from build123d import *

# Parameters (mm, degrees)
ESTRUSIONE_ESTRUSIONE1_DEPTH = 20
TAGLIO_ESTRUSIONE1_REACH     = 37.979
ESTRUSIONE_ESTRUSIONE4_DEPTH = 0.6
SCHIZZO12_W                  = 2
SCHIZZO12_H                  = 6
TAGLIO_ESTRUSIONE2_DEPTH     = 11


with BuildPart() as part:
    # Schizzo2 → Estrusione-Estrusione1 (new body)
    with BuildSketch(Plane.XY):
        with BuildLine():
            Line((-4, 9.5), (-11, 9.5))
            Line((-11, 9.5), (-11, 23.5))
            Line((-11, 23.5), (-6, 23.5))
            ThreePointArc((-6, 23.5), (-5.292893219, 23.207106781), (-5, 22.5))
            Line((-5, 22.5), (-5, 12.5))
            Line((-5, 12.5), (4, 12.5))
            Line((4, 12.5), (4, 9.5))
            Line((4, 9.5), (4, 6.5))
            Line((4, 6.5), (7.5, 6.5))
            Line((7.5, 6.5), (7.5, 4))
            Line((7.5, 4), (4, 0))
            Line((4, 0), (-4, 0))
            Line((-4, 0), (-7.5, 4))
            Line((-7.5, 4), (-7.5, 6.5))
            Line((-7.5, 6.5), (-4, 6.5))
            Line((-4, 6.5), (-4, 9.5))
        make_face()
    extrude(amount=-ESTRUSIONE_ESTRUSIONE1_DEPTH)

    # Schizzo6 → Taglio-Estrusione1 (cut, up to next)
    with BuildSketch(Plane.ZY.offset(11), mode=Mode.PRIVATE) as taglio_estrusione1_sk1:
        with BuildLine():
            Line((-8.5, 20), (-8.5, 17))
            ThreePointArc((-8.5, 17), (-10, 15.5), (-11.5, 17))
            Line((-11.5, 17), (-11.5, 20))
            ThreePointArc((-11.5, 20), (-10, 21.5), (-8.5, 20))
        make_face()
    taglio_estrusione1_tool1 = extrude(taglio_estrusione1_sk1.sketch, amount=-TAGLIO_ESTRUSIONE1_REACH, mode=Mode.PRIVATE) & part.part
    add(taglio_estrusione1_tool1.solids().sort_by_distance((-11, 18.5, -10))[0], mode=Mode.SUBTRACT)

    # Schizzo11 → Estrusione-Estrusione4 (add)
    with BuildSketch(Plane(origin=(0, 0, -20), x_dir=(-1, 0, 0), z_dir=(0, 0, -1))):
        with BuildLine():
            Line((-1.916666667, 6), (-2.5, 6))
            add(Edge.make_bspline(
                [(-2.5, 6), (-2.484196549, 6.065431756), (-2.453302094, 6.193345487), (-2.388863743, 6.376101829), (-2.318665127, 6.549045511), (-2.234371075, 6.708938219), (-2.142426246, 6.858993324), (-2.037084049, 6.995807413), (-1.923204564, 7.122860063), (-1.797243944, 7.235613218), (-1.665147858, 7.337714716), (-1.525054993, 7.424768393), (-1.379783905, 7.499656106), (-1.228328086, 7.561350822), (-1.070236625, 7.607826795), (-0.906938753, 7.641546577), (-0.738006538, 7.66344436), (-0.623332441, 7.665581492), (-0.565104167, 7.666666667)],
                knots=[0, 0, 0, 0, 1.162005537, 2.271625781, 3.343758855, 4.383309926, 5.390229558, 6.379919256, 7.361854164, 8.333198761, 9.295911338, 10.242430842, 11.177959212, 12.116337295, 13.062827104, 14.020064771, 14.994644689, 16, 16, 16, 16], degree=3))
            add(Edge.make_bspline(
                [(-0.565104167, 7.666666667), (-0.480264789, 7.664105239), (-0.312436625, 7.659038256), (-0.065876681, 7.612768588), (0.171887412, 7.539550485), (0.398253158, 7.438384992), (0.608515961, 7.313608553), (0.795597451, 7.165102613), (0.956961828, 6.995732482), (1.092337101, 6.80865772), (1.198333527, 6.608726059), (1.276493935, 6.402954339), (1.324077057, 6.191830678), (1.330243806, 6.049281445), (1.333333333, 5.977864583)],
                knots=[0, 0, 0, 0, 1.083050992, 2.142477498, 3.193116406, 4.255571735, 5.30263384, 6.308962982, 7.297363603, 8.282367274, 9.249857812, 10.179914175, 11.08814088, 12, 12, 12, 12], degree=3))
            add(Edge.make_bspline(
                [(1.333333333, 5.977864583), (1.331172379, 5.909137679), (1.326943725, 5.774649792), (1.291038272, 5.578309869), (1.230613784, 5.393261183), (1.146912796, 5.218724739), (1.038564203, 5.055807179), (0.907314909, 4.904141953), (0.752238537, 4.763056374), (0.634720509, 4.682234495), (0.57421875, 4.640625)],
                knots=[0, 0, 0, 0, 1.024540389, 2.004866551, 2.965041327, 3.920577974, 4.882998113, 5.874504559, 6.905732034, 8, 8, 8, 8], degree=3))
            add(Edge.make_bspline(
                [(0.57421875, 4.640625), (0.643363437, 4.607236967), (0.780359061, 4.541085617), (0.967095758, 4.411353496), (1.136611813, 4.261563137), (1.231147291, 4.144669639), (1.278645833, 4.0859375)],
                knots=[0, 0, 0, 0, 1.015518401, 2.012035669, 3.001164323, 4, 4, 4, 4], degree=3))
            add(Edge.make_bspline(
                [(1.278645833, 4.0859375), (1.309922612, 4.043115961), (1.37196399, 3.958174116), (1.448544267, 3.821606468), (1.518018337, 3.683525131), (1.572154458, 3.540229091), (1.614077354, 3.393379209), (1.644044271, 3.24272333), (1.662660533, 3.088138431), (1.665326558, 2.983558111), (1.666666667, 2.930989583)],
                knots=[0, 0, 0, 0, 1.025084078, 2.033381695, 3.024893161, 4.013698104, 4.991890475, 5.976764909, 6.982997093, 8, 8, 8, 8], degree=3))
            add(Edge.make_bspline(
                [(1.666666667, 2.930989583), (1.663333999, 2.83997153), (1.656684346, 2.658363755), (1.597248208, 2.390053558), (1.505109333, 2.127777625), (1.374260737, 1.876924352), (1.214792507, 1.64221793), (1.025071762, 1.43221907), (0.807254146, 1.251707377), (0.56432937, 1.100888382), (0.301140417, 0.980326526), (0.019642889, 0.896648418), (-0.276107211, 0.842148704), (-0.478920764, 0.836304519), (-0.58203125, 0.833333333)],
                knots=[0, 0, 0, 0, 0.955779014, 1.907060117, 2.875433937, 3.871313158, 4.872415639, 5.851225146, 6.836215519, 7.83643374, 8.849228613, 9.86973379, 10.916971861, 12, 12, 12, 12], degree=3))
            add(Edge.make_bspline(
                [(-0.58203125, 0.833333333), (-0.651524236, 0.834945729), (-0.78826326, 0.838118387), (-0.9892869, 0.859807218), (-1.181170056, 0.899420085), (-1.364172166, 0.952726223), (-1.538455805, 1.020310887), (-1.703489143, 1.104474184), (-1.860287517, 1.203481259), (-2.007371283, 1.318500779), (-2.144722909, 1.447166124), (-2.268692254, 1.591761428), (-2.381346155, 1.74961375), (-2.479668199, 1.922556569), (-2.568136825, 2.108354904), (-2.640901459, 2.309387829), (-2.704946086, 2.523858156), (-2.73472252, 2.673316816), (-2.75, 2.75)],
                knots=[0, 0, 0, 0, 1.048658725, 2.063410685, 3.046034179, 4.001477787, 4.936774919, 5.862367409, 6.792675028, 7.730719943, 8.675894397, 9.627829632, 10.600096036, 11.597688215, 12.626045268, 13.701542398, 14.82072376, 16, 16, 16, 16], degree=3))
            Line((-2.75, 2.75), (-2.166666667, 2.75))
            add(Edge.make_bspline(
                [(-2.166666667, 2.75), (-2.151469125, 2.699951833), (-2.121908588, 2.602603799), (-2.071590606, 2.462500375), (-2.014263815, 2.33406399), (-1.952765349, 2.216352478), (-1.888176806, 2.108206588), (-1.815906231, 2.012485974), (-1.74130639, 1.924986312), (-1.685073305, 1.875689176), (-1.657552083, 1.8515625)],
                knots=[0, 0, 0, 0, 1.198163088, 2.33053128, 3.407730985, 4.417276592, 5.372219308, 6.28897303, 7.162600585, 8, 8, 8, 8], degree=3))
            add(Edge.make_bspline(
                [(-1.657552083, 1.8515625), (-1.621158441, 1.823504166), (-1.548483496, 1.767474107), (-1.430056781, 1.695971082), (-1.305507707, 1.634014892), (-1.172137598, 1.586688029), (-1.032824452, 1.54661523), (-0.885316488, 1.520391409), (-0.730915085, 1.502399091), (-0.625489239, 1.500811361), (-0.571614583, 1.5)],
                knots=[0, 0, 0, 0, 0.946170439, 1.889420265, 2.845303464, 3.807233317, 4.801018734, 5.828864929, 6.890507805, 8, 8, 8, 8], degree=3))
            add(Edge.make_bspline(
                [(-0.571614583, 1.5), (-0.51078665, 1.501143824), (-0.391842877, 1.503380473), (-0.218283853, 1.523949643), (-0.053170021, 1.553906125), (0.101665412, 1.600173093), (0.24825064, 1.657337532), (0.384530847, 1.729113142), (0.512295044, 1.813324768), (0.629906797, 1.909040348), (0.735662739, 2.013823125), (0.828778978, 2.123418828), (0.907939064, 2.237365369), (0.97179428, 2.356293307), (1.022216731, 2.479710161), (1.056542675, 2.607962273), (1.080409774, 2.740000053), (1.082353483, 2.829753852), (1.083333333, 2.875)],
                knots=[0, 0, 0, 0, 1.217147791, 2.380027433, 3.494444702, 4.572153297, 5.609568379, 6.639424714, 7.649109417, 8.668170816, 9.669597737, 10.625200337, 11.543417969, 12.441394052, 13.322311151, 14.205496177, 15.095365482, 16, 16, 16, 16], degree=3))
            add(Edge.make_bspline(
                [(1.083333333, 2.875), (1.080491345, 2.935563915), (1.074821509, 3.056390388), (1.031534147, 3.234151597), (0.960333399, 3.405423649), (0.860655878, 3.567284402), (0.739318097, 3.71729679), (0.597497555, 3.851143829), (0.43401656, 3.961588284), (0.283551089, 4.037895789), (0.150272941, 4.089964642), (0.036215798, 4.124646719), (-0.091475036, 4.154014937), (-0.231255399, 4.181337727), (-0.384178515, 4.204591659), (-0.5500779, 4.223983603), (-0.728987171, 4.239500107), (-0.852842194, 4.246429284), (-0.916666667, 4.25)],
                knots=[0, 0, 0, 0, 1.07054697, 2.135767047, 3.216561865, 4.33974944, 5.486079747, 6.621378074, 7.775625952, 8.963672916, 9.598146892, 10.304877434, 11.070270905, 11.915000392, 12.823868403, 13.805723172, 14.86925407, 16, 16, 16, 16], degree=3))
            Line((-0.916666667, 4.25), (-0.916666667, 4.916666667))
            add(Edge.make_bspline(
                [(-0.916666667, 4.916666667), (-0.836250216, 4.918031302), (-0.678734144, 4.920704288), (-0.448644721, 4.95303345), (-0.228622855, 4.997754616), (-0.02354462, 5.066255688), (0.163374419, 5.145816239), (0.325539394, 5.238398914), (0.460678382, 5.34131202), (0.568134658, 5.456144008), (0.648974654, 5.579300525), (0.708081563, 5.707660032), (0.742996455, 5.842347574), (0.747657265, 5.934266243), (0.75, 5.98046875)],
                knots=[0, 0, 0, 0, 1.321986639, 2.589447074, 3.816329219, 5.01088745, 6.139805852, 7.153945165, 8.075214402, 8.924034688, 9.728124013, 10.488707548, 11.240355623, 12, 12, 12, 12], degree=3))
            add(Edge.make_bspline(
                [(0.75, 5.98046875), (0.74923038, 6.014413134), (0.747699256, 6.081943876), (0.728390026, 6.180604717), (0.69937395, 6.276249331), (0.659483024, 6.368470979), (0.606089798, 6.456630059), (0.542192966, 6.541478178), (0.466109351, 6.622530911), (0.37892495, 6.698080076), (0.285303026, 6.770080088), (0.182696301, 6.831205413), (0.074198534, 6.883474814), (-0.040310397, 6.926578176), (-0.161202096, 6.959002568), (-0.28790856, 6.982283416), (-0.420671401, 6.996839061), (-0.511247475, 6.99893469), (-0.557291667, 7)],
                knots=[0, 0, 0, 0, 0.884392785, 1.759457502, 2.611959086, 3.489218968, 4.37281399, 5.2945488, 6.255912374, 7.266815255, 8.301784654, 9.332968512, 10.37626691, 11.440494194, 12.520033166, 13.637162961, 14.798855837, 16, 16, 16, 16], degree=3))
            add(Edge.make_bspline(
                [(-0.557291667, 7), (-0.631301907, 6.997416042), (-0.775861121, 6.992368971), (-0.984260252, 6.948163375), (-1.177996158, 6.877632648), (-1.326082253, 6.793442755), (-1.435435605, 6.710334806), (-1.51357849, 6.637753232), (-1.590316581, 6.557092273), (-1.660601409, 6.463383862), (-1.731681652, 6.362974109), (-1.79639298, 6.2507587), (-1.859275266, 6.129664825), (-1.897165715, 6.044058647), (-1.916666667, 6)],
                knots=[0, 0, 0, 0, 1.472543308, 2.876219568, 4.221790263, 5.565193594, 6.249813518, 6.953379497, 7.687249741, 8.463570142, 9.283606569, 10.136032583, 11.040678096, 12, 12, 12, 12], degree=3))
        make_face()
    extrude(amount=ESTRUSIONE_ESTRUSIONE4_DEPTH)

    # Schizzo12 → Taglio-Estrusione2 (cut)
    with BuildSketch(Plane(origin=(0, 23.5, 0), x_dir=(1, 0, 0), z_dir=(0, 1, 0))):
        with Locations((-8.5, 10)):
            Rectangle(SCHIZZO12_W, SCHIZZO12_H)
    extrude(amount=-TAGLIO_ESTRUSIONE2_DEPTH, mode=Mode.SUBTRACT)


solid = part.part
The model under review builds one solid part; all positions refer to its coordinate system, in mm. A direction names the side the tool comes from. Round coordinates to 2 decimals unless told otherwise and drop trailing zeros. Order: outer loops, then holes, each group sorted by start corner. A loop starts at its lowest first (then second) coordinate and runs counter-clockwise, first axis right, second up. Notation, with made-up numbers: (-23, 73) -> (2, 73) arc R7 ccw to (2, 77) -> close; hole circle Ø6 at (49, 56.25). An arc over 180 degrees is marked (long way). Write item = value, one per line. Start each with the question number.
Item 1: Consider section B-B on x = -4.5. Write out the cut boundary in (y, z), plus the area to 3 significant figures.
Item 2: Mouldability with a two-part tool opening along X and no side actions: class faces 1 (the face through (-10, 23.5, -10)), 2 (the face through (-7.5, 18, -12)), 3 (the face through (-5.726, 1.972, -9.86)) as released by +X, released by -X, zero draft, split by the parting line, or undercut.
Item 3: For line 1 along X through (y, z) = (21.25, -8); line 2 along Y through (x, z) = (-5.25, -9.5); line 3 along X through (y, z) = (4.5, -8.5), list the stretches that pass through material, from the lowest coordinate up.
Item 4: For faces 4 (the face through (-7.5, 5, -10)), 5 (the face through (-4, 8, -10)), 6 (the face through (-9, 18, -13)), 7 (the face through (-1, 12.5, -10)), 8 (the face through (-6, 18, -11.5)), list the 3-axis set-ups (+Z, -Z, +X, -X, +Y, -Y) from which the entire face can be reached by the end or side of a thin tool; tool diameter is ignored.
Item 5: Clearance check with flat-ended pins moving along their axes: pin 1 Ø5 at (y, z) = (17, -8.5) entering from +X; pin 2 Ø5 at (x, y) = (-6, 6) entering from -Z; pin 3 Ø3 at (x, z) = (6, -12) entering from +Y. State where each tip first meets the part, or that it passes through.
Item 6: Consider section C-C on y = 16.5. Write out the cut boundary in (x, z).
Item 7: Consider section A-A on z = -10. Write out the cut boundary in (x, y), plus the area to 3 significant figures.
Item 8: Consider section D-D on z = -12.5. Write out the cut boundary in (x, y), plus the area to 3 significant figures.
Conclusion:
q1.outline = (0.57, -20) -> (6.5, -20) -> (6.5, 0) -> (0.57, 0) -> close; (9.5, -20) -> (12.5, -20) -> (12.5, 0) -> (9.5, 0) -> close
q1.area = 179 mm2
q2.face_1 = zero draft
q2.face_2 = undercut
q2.face_3 = released by -X
q3.line_1 = -11 to -9.5, -7.5 to -5
q3.line_2 = 1.43 to 6.5, 9.5 to 15.59, 21.41 to 23.16
q3.line_3 = -7.5 to 7.5
q4.face_4 = +Z, -Z, -X, -Y
q4.face_5 = +Z, -Z, -X
q4.face_6 = +Y
q4.face_7 = +Z, -Z, +X, +Y
q4.face_8 = +X, -X
q5.pin_1 = -5
q5.pin_2 = -20
q5.pin_3 = 6.5
q6.outline = (-11, -20) -> (-5, -20) -> (-5, -11.41) -> (-7.5, -11.41) -> (-7.5, -13) -> (-9.5, -13) -> (-9.5, -11.41) -> (-11, -11.41) -> close; (-11, -8.59) -> (-9.5, -8.59) -> (-9.5, -7) -> (-7.5, -7) -> (-7.5, -8.59) -> (-5, -8.59) -> (-5, 0) -> (-11, 0) -> close
q7.outline = (-11, 9.5) -> (-4, 9.5) -> (-4, 6.5) -> (-7.5, 6.5) -> (-7.5, 4) -> (-4, 0) -> (4, 0) -> (7.5, 4) -> (7.5, 6.5) -> (4, 6.5) -> (4, 12.5) -> (-5, 12.5) -> (-5, 15.5) -> (-7.5, 15.5) -> (-7.5, 12.5) -> (-9.5, 12.5) -> (-9.5, 15.5) -> (-11, 15.5) -> close; (-11, 21.5) -> (-9.5, 21.5) -> (-9.5, 23.5) -> (-11, 23.5) -> close; (-7.5, 21.5) -> (-5, 21.5) -> (-5, 22.5) arc R1 ccw to (-6, 23.5) -> (-7.5, 23.5) -> close
q7.area = 172 mm2
q8.outline = (-11, 9.5) -> (-4, 9.5) -> (-4, 6.5) -> (-7.5, 6.5) -> (-7.5, 4) -> (-4, 0) -> (4, 0) -> (7.5, 4) -> (7.5, 6.5) -> (4, 6.5) -> (4, 12.5) -> (-5, 12.5) -> (-5, 22.5) arc R1 ccw to (-6, 23.5) -> (-7.5, 23.5) -> (-7.5, 12.5) -> (-9.5, 12.5) -> (-9.5, 23.5) -> (-11, 23.5) -> close
q8.area = 196 mm2
